Read the model definition and answer for the solid it produces. Units are mm, in the model's axes. A direction names the side the tool comes from. Coordinates: 2 decimals unless noted, no trailing zeros. Loops run counter-clockwise (first coordinate to the right, second up) from the corner with the lowest first, then second, coordinate; pieces in that order, holes last. Notation, with made-up numbers: (79, -22.5) - (107, -22.5) arc R8 ccw to (107, -9.5) - close; hole circle Ø6 at (-29.5, 74.5). An arc over 180 degrees is marked (long way). Use CSV: the item, a comma, the result in double quotes.
```python
from build123d import *

# Parameters (mm, degrees)
SKETCH2_W           = 24.8
SKETCH2_H           = 16
SKETCH2_W_2         = 3
SKETCH2_H_2         = 12.75
BOSS_EXTRUDE1_DEPTH = 5.15
BOSS_EXTRUDE2_DEPTH = 5


with BuildPart() as part:
    # Sketch2 → Boss-Extrude1 (new body)
    with BuildSketch(Plane(origin=(0, 0, 0), x_dir=(1, 0, 0), z_dir=(0, 1, 0))):
        with Locations((12.4, -8)):
            Rectangle(SKETCH2_W, SKETCH2_H)
        with Locations((21.2, -8)):
            Rectangle(SKETCH2_W_2, SKETCH2_H_2, mode=Mode.SUBTRACT)
    extrude(amount=BOSS_EXTRUDE1_DEPTH)

    # Sketch4 → Boss-Extrude2 (add)
    with BuildSketch(Plane(origin=(0, 5.15, 0), x_dir=(1, 0, 0), z_dir=(0, 1, 0))):
        Polygon((2.1, -1.625), (19.7, -1.625), (22.7, -1.625), (24.8, -1.625), (24.8, 0), (0, 0), (0, -16), (24.8, -16), (24.8, -14.375), (22.7, -14.375), (19.7, -14.375), (2.1, -14.375), align=None)
    extrude(amount=BOSS_EXTRUDE2_DEPTH)


solid = part.part
```
Q1. The part is cut by section A-A on y = 3. Determine the outline of the cut face in (x, z) (3 decimals).
Reported:
outline,"(0, 0) - (24.8, 0) - (24.8, 16) - (0, 16) - close; hole (19.7, 1.625) - (22.7, 1.625) - (22.7, 14.375) - (19.7, 14.375) - close"
Q2. Find the intervals of material crossed by probe 1 along Z at (x, y) = (7.75, 8.5) (3 decimals); probe 2 along X at (y, z) = (1.5, 4.75); probe 3 along X at (y, z) = (6.25, 3.5), in increasing order. Write a range as [from, to].
Reported:
probe 1,"z = [0, 1.625], [14.375, 16]"
probe 2,"x = [0, 19.7], [22.7, 24.8]"
probe 3,"x = [0, 2.1]"
Q3. The part is cut by section D-D on x = 10.5. Determine the outline of the cut face in (y, z) (3 decimals).
Reported:
outline,"(0, 0) - (10.15, 0) - (10.15, 1.625) - (5.15, 1.625) - (5.15, 14.375) - (10.15, 14.375) - (10.15, 16) - (0, 16) - close"
Q4. The part is cut by section B-B on z = 5. Determine the outline of the cut face in (x, y), and give its area (3 significant figures).
Reported:
outline,"(0, 0) - (19.7, 0) - (19.7, 5.15) - (2.1, 5.15) - (2.1, 10.15) - (0, 10.15) - close; (22.7, 0) - (24.8, 0) - (24.8, 5.15) - (22.7, 5.15) - close"
area,"123 mm²"
Q5. Given P1, Ø1.5, axis at x = 7, z = 4.5, coming from the -Y side; P2, Ø0.6, axis at x = 24, z = 11, coming from the +Y side, each flat-ended and moving along its own axis, determine where each tip first touches the part or whether it passes through.
Reported:
P1,"stops at y = 0"
P2,"stops at y = 5.15"
Q6. The part is cut by section C-C on y = 8. Determine the outline of the cut face in (x, z) (3 decimals), and give its area (3 significant figures).
Reported:
outline,"(0, 0) - (24.8, 0) - (24.8, 1.625) - (2.1, 1.625) - (2.1, 14.375) - (24.8, 14.375) - (24.8, 16) - (0, 16) - close"
area,"107 mm²"
Q7. A tool of negligible diameter and unlimited length cuts with its end or side. For faces 1 (the face through (13, 7, 1.625)), 2 (the face through (13, 5, 0)), 3 (the face through (24, 5.15, 8)), 4 (the face through (22.7, 3, 8)), 5 (the face through (12, 0, 8)), from which of +Z, -Z, +X, -X, +Y, -Y can it reach the whole face along a straight path? Write none if from no direction.
Reported:
face 1,"+Y"
face 2,"-Z, +X, -X, +Y, -Y"
face 3,"+X, +Y"
face 4,"+Y, -Y"
face 5,"+Z, -Z, +X, -X, -Y"
